from build123d import *

# Parameters (mm, degrees)
SKETCH_1_W          = 8.5
SKETCH_1_H          = 5
SKETCH_2_R          = 1.6
CUT_EXTRUDE_1_DEPTH = 27.43066401
SKETCH_3_R          = 1.6
CUT_EXTRUDE_2_DEPTH = 27.430664048


with BuildPart() as part:
    # ｽｹｯﾁ1 → 回転2 (revolve)
    with BuildSketch(Plane.XY, mode=Mode.PRIVATE) as revolve_2_sk:
        Polygon((-4, 0), (-4, 5), (-12.5, 5), (-15, 5), (-15, 2.5), (-17.3, 2.5), (-17.3, 0), align=None)
        with Locations((-8.25, 7.5)):
            Rectangle(SKETCH_1_W, SKETCH_1_H)
    revolve(revolve_2_sk.sketch.rotate(Axis((0, 0, 0), (0, 1, 0)), 270), axis=Axis((0, 0, 0), (0, 1, 0)))

    # ｽｹｯﾁ2 → ｶｯﾄ - 押し出し1 (cut, through all)
    with BuildSketch(Plane.XY):
        with Locations(Location((0, 7.5, 0), (0, 0, 90))):
            Circle(SKETCH_2_R)
    extrude(amount=-CUT_EXTRUDE_1_DEPTH, mode=Mode.SUBTRACT)

    # ｽｹｯﾁ3 → ｶｯﾄ - 押し出し2 (cut, through all)
    with BuildSketch(Plane(origin=(0, 10, 0), x_dir=(1, 0, 0), z_dir=(0, 1, 0))):
        with Locations(Location((-9, 0, 0), (0, 0, 270))):
            Circle(SKETCH_3_R)
    extrude(amount=-CUT_EXTRUDE_2_DEPTH, mode=Mode.SUBTRACT)


solid = part.part
For this review, take the finished solid that the model builds, in its own axes (mm). A direction names the side the tool comes from. Give positions to 0.01 mm unless a question says otherwise; leave off trailing zeros. Order: outer loops, then holes, each group sorted by start corner. A loop starts at its lowest first (then second) coordinate and runs counter-clockwise, first axis right, second up. Notation, with made-up numbers: (13, -26.75) - (36, -26.75) arc R24 cw to (36, 0.25) - close; hole circle Ø5 at (68, 8.5). An arc over 180 degrees is marked (long way). Answer as a JSON object with one key per item and string values. Group by question number.
Item 1: Take a section at C-C on x = 0. Give the boundary of the cut face in (y, z), and give its area (3 significant figures).
Item 2: Take a section at A-A on x = -9. Give the boundary of the cut face in (y, z), and give its area (3 significant figures).
Item 3: Take a section at B-B on z = 0. Give the boundary of the cut face in (x, y), and give its area (4 significant figures).
Item 4: Clearance check with flat-ended pins moving along their axes: pin 1 Ø1.5 at (x, y) = (5, 5.5) entering from -Z; pin 2 Ø3.5 at (x, y) = (0, 7.5) entering from +Z; pin 3 Ø5 at (y, z) = (6, 1.5) entering from +X. State where each tip first meets the part, or that it passes through.
Item 5: Machinability: for faces 4 (the flat face through (-12.3, 5, -3.4)), 5 (the cylindrical face through (-0.07, 5.9, -8.02)), 6 (the cylindrical face through (0, 5, 4)), which of the approach directions +Z, -Z, +X, -X, +Y, -Y give a long, thin tool a straight path to every point of the face, cutting with its end or side? Answer none if there is none.
Item 6: Take a section at D-D on y = 1.5. Give the boundary of the cut face in (x, z), and give its area (3 significant figures).
Item 7: Draft analysis for pull direction X (two halves, no side actions). For faces 1 (the cylindrical face through (-10.56, 5.07, -0.35)), 2 (the cylindrical face through (-0.66, 3.732, 14.985)), 3 (the flat face through (4, 0, -4)), state which applies: pulls with the +X half, pulls with the -X half, needs draft (parallel to the pull), parting line crosses it, or undercut.
Item 8: Wall thickness on line 1 along X through (y, z) = (3.5, 0); line 2 along X through (y, z) = (6.25, 0); line 3 along Y through (x, z) = (16.5, 4): over which ranges is each line inside the solid? List them lowest first.
Reported:
{
 "1": {"outline": "(0, -17.3) - (2.5, -17.3) - (2.5, -15) - (5, -15) - (5, -12.5) - (5.9, -12.5) - (5.9, -4) - (0, -4) - close; (0, 4) - (10, 4) - (10, 12.5) - (5, 12.5) - (5, 15) - (2.5, 15) - (2.5, 17.3) - (0, 17.3) - close; (9.1, -12.5) - (10, -12.5) - (10, -4) - (9.1, -4) - close", "area": "179 mm^2"},
 "2": {"outline": "(0, -14.77) - (2.5, -14.77) - (2.5, -12) - (5, -12) - (5, -8.67) - (10, -8.67) - (10, -1.6) - (0, -1.6) - close; (0, 1.6) - (10, 1.6) - (10, 8.67) - (5, 8.67) - (5, 12) - (2.5, 12) - (2.5, 14.77) - (0, 14.77) - close", "area": "189 mm^2"},
 "3": {"outline": "(-17.3, 0) - (-10.6, 0) - (-10.6, 10) - (-12.5, 10) - (-12.5, 5) - (-15, 5) - (-15, 2.5) - (-17.3, 2.5) - close; (-7.4, 0) - (-4, 0) - (-4, 10) - (-7.4, 10) - close; (4, 0) - (17.3, 0) - (17.3, 2.5) - (15, 2.5) - (15, 5) - (12.5, 5) - (12.5, 10) - (4, 10) - close", "area": "174.5 mm^2"},
 "4": {"pin 1": "z = -14.33", "pin 2": "z = 12.5", "pin 3": "x = 15"},
 "5": {"face 4": "+Y", "face 5": "-Z", "face 6": "+Y, -Y"},
 "6": {"outline": "circle Ø34.6 at (0, 0); hole circle Ø3.2 at (-9, 0); hole circle Ø8 at (0, 0)", "area": "882 mm^2"},
 "7": {"face 1": "undercut", "face 2": "parting line crosses it", "face 3": "needs draft"},
 "8": {"line 1": "-15 to -10.6, -7.4 to -4, 4 to 15", "line 2": "-12.5 to -10.6, -7.4 to -4, 4 to 12.5", "line 3": "0 to 2.5"}
}
